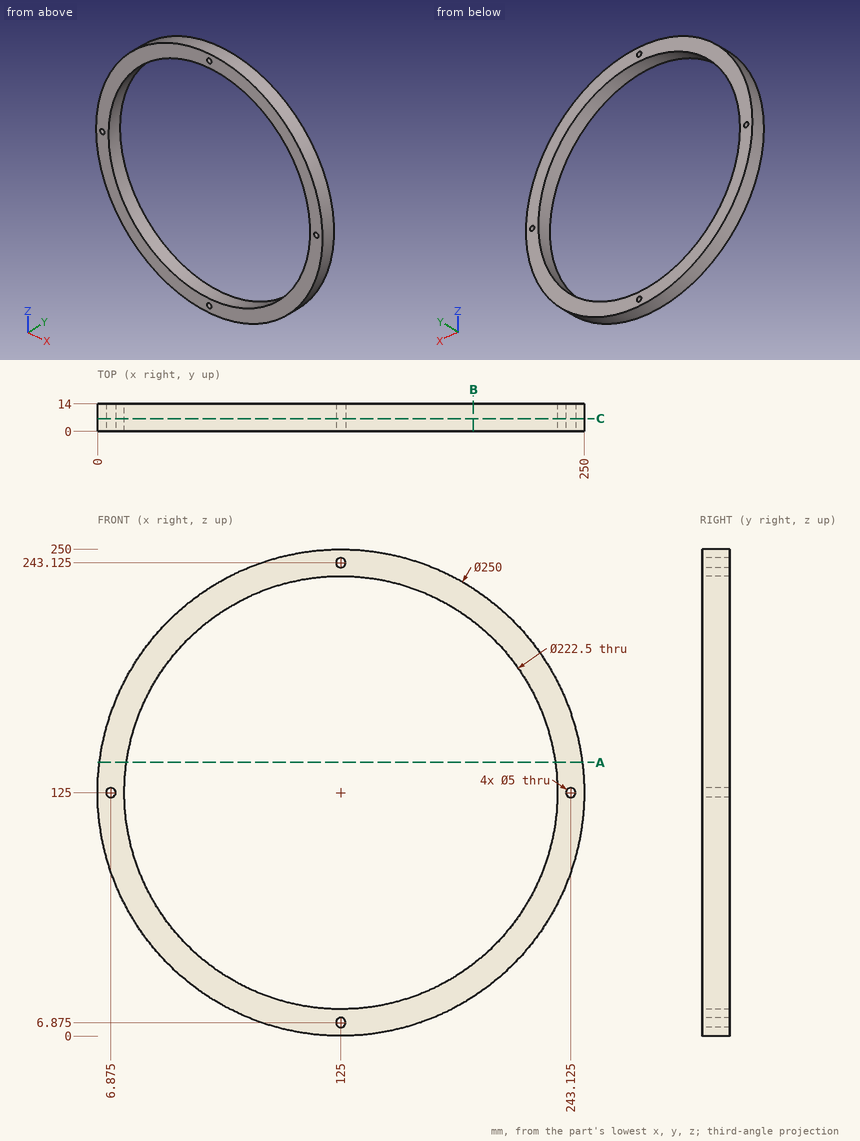
For this review, use the dimensioned drawing (mm, ordinates from the lowest corner) and the shaded views. Coordinates: 2 decimals unless noted, no trailing zeros. Loops run counter-clockwise (first coordinate to the right, second up) from the corner with the lowest first, then second, coordinate; pieces in that order, holes last. Notation, with made-up numbers: (59.5, -31) -> (79.5, -31) arc R9 cw to (79.5, -23) -> close; hole circle Ø4 at (-11.5, 48.5). An arc over 180 degrees is marked (long way). Write each question's results on one line, items separated by ' | '.
Q1. Add section B-B, the plane x = 193. State the section outline as (y, z) points.
Taken from the geometry:
outline: (0, 20.11) -> (14, 20.11) -> (14, 36.95) -> (0, 36.95) -> close; (0, 213.05) -> (14, 213.05) -> (14, 229.89) -> (0, 229.89) -> close
Q2. Add section C-C, the plane y = 6.5. State the section outline as (x, z) points (3 decimals).
Taken from the geometry:
outline: circle Ø250 at (125, 125); hole circle Ø5 at (6.875, 125); hole circle Ø222.5 at (125, 125); hole circle Ø5 at (125, 6.875); hole circle Ø5 at (125, 243.125); hole circle Ø5 at (243.125, 125)
Q3. To check wall thickness, follow line 1 along Z through (x, y) = (128, 1.75); line 2 along X through (y, z) = (7.5, 121.5); line 3 along X through (y, z) = (1.5, 119). State the ranges of each line that lie inside material, in increasing order. Write a range as [from, to].
Taken from the geometry:
line 1: [0.04, 13.79], [236.21, 249.96] | line 2: [0.05, 13.81], [236.19, 249.95] | line 3: [0.14, 13.91], [236.09, 249.86]
Q4. Add section A-A, the plane z = 140.5. State the section outline as (x, y) points, then the cut area to 3 significant figures.
Taken from the geometry:
outline: (0.96, 0) -> (14.84, 0) -> (14.84, 14) -> (0.96, 14) -> close; (235.16, 0) -> (249.04, 0) -> (249.04, 14) -> (235.16, 14) -> close | area: 388 mm²
Q5. For pin 1 Ø1 at (x, y) = (204.5, 5) entering from +Z; pin 2 Ø3 at (x, z) = (125, 243.125) entering from +Y; pin 3 Ø6 at (x, y) = (73, 1.5) entering from +Z; pin 4 Ø5 at (x, y) = (67.5, 6) entering from +Z, all flat-tipped, find the tip position at first contact; note any pin that passes through.
Taken from the geometry:
pin 1: z = 221.87 | pin 2: through | pin 3: z = 240 | pin 4: z = 237.25
